```python
from build123d import *

# Parameters (mm, degrees)
SKETCH1_R           = 25
BOSS_EXTRUDE1_DEPTH = 20
SKETCH2_R           = 5
BOSS_EXTRUDE2_DEPTH = 10
SKETCH3_R           = 10
CUT_EXTRUDE1_DEPTH  = 41.620192023
CUT_EXTRUDE2_START  = -9
SKETCH5_R           = 25
SKETCH5_R_2         = 22.5
CUT_EXTRUDE2_DEPTH  = 8


with BuildPart() as part:
    # Sketch1 → Boss-Extrude1 (new body)
    with BuildSketch(Plane.XY):
        Circle(SKETCH1_R)
    extrude(amount=BOSS_EXTRUDE1_DEPTH)

    # Sketch2 → Boss-Extrude2 (add)
    with BuildSketch(Plane(origin=(0, 0, 0), x_dir=(-1, 0, 0), z_dir=(0, 0, -1))):
        with Locations(Location((0, -20, 0), (0, 0, 270))):
            Circle(SKETCH2_R)
    extrude(amount=BOSS_EXTRUDE2_DEPTH)

    # Sketch3 → Cut-Extrude1 (cut, through all)
    with BuildSketch(Plane(origin=(0, 0, 0), x_dir=(-1, 0, 0), z_dir=(0, 0, -1))):
        Circle(SKETCH3_R)
    extrude(amount=-CUT_EXTRUDE1_DEPTH, mode=Mode.SUBTRACT)

    # Sketch5 → Cut-Extrude2 (cut)
    with BuildSketch(Plane.XY.offset(20).offset(CUT_EXTRUDE2_START)):
        with Locations(Location((0, 0, 0), (0, 0, 270))):
            Circle(SKETCH5_R)
        Circle(SKETCH5_R_2, mode=Mode.SUBTRACT)
    extrude(amount=CUT_EXTRUDE2_DEPTH, mode=Mode.SUBTRACT)


solid = part.part
```
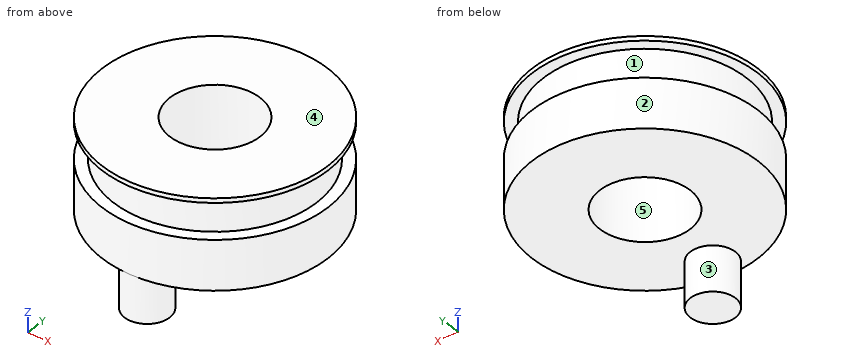
Geometry check sheet. Reference: the model listing, model coordinates, mm. Face numbers are marked on the shaded views. A direction names the side the tool comes from. Coordinates: 2 decimals unless noted, no trailing zeros. Order: outer loops, then holes, each group sorted by start corner. A loop starts at its lowest first (then second) coordinate and runs counter-clockwise, first axis right, second up. Notation, with made-up numbers: (-32.5, 82.5) - (9.5, 82.5) arc R33 cw to (9.5, 121.5) - close; hole circle Ø11 at (11, 18). An arc over 180 degrees is marked (long way). Use one line per item in the form item = value.
1. Section check D-D (x = 15). Record the boundary of the cut face in (y, z), then the cut area to 3 significant figures.
Here are the results:
outline = (-20, 0) - (20, 0) - (20, 11) - (16.77, 11) - (16.77, 19) - (20, 19) - (20, 20) - (-20, 20) - (-20, 19) - (-16.77, 19) - (-16.77, 11) - (-20, 11) - close
area = 748 mm²
2. Access from +Z, -Z, +X, -X, +Y, -Y to the whole of each face (thin tool, end or side, straight path). Record for the marked faces 1 and 2.
Here are the results:
face_1 = none
face_2 = +Z, -Z
3. Scan lines: line 1 (Y direction, x = 0, z = 7.25); line 2 (Z direction, x = -16.5, y = -15.5); line 3 (Z direction, x = -11.5, y = -9.5). Record each from-to range of solid material in increasing order.
Here are the results:
line_1 = -25 to -10, 10 to 25
line_2 = 0 to 11, 19 to 20
line_3 = 0 to 20
4. Draft check along Y on the marked faces 3, 4 and 5. Enter one of: pulls with the +Y half, pulls with the -Y half, needs draft (parallel to the pull), parting line crosses it, or undercut.
Here are the results:
face_3 = parting line crosses it
face_4 = needs draft
face_5 = undercut
5. Gauge pin test, flat ends, axial feed: pin 1 (3 mm diameter, centred on x = 8, z = 8.5, fed in from +Y); pin 2 (1.5 mm diameter, centred on y = 13.5, z = 12, fed in from +X); pin 3 (6 mm diameter, centred on y = -5.5, z = 15, fed in from -X). Record the tip position at first contact, or that the pin passes through.
Here are the results:
pin_1 = 24.14
pin_2 = 18.54
pin_3 = -22.36
6. Section check C-C (z = 3.25). Record the boundary of the cut face in (x, y), then the cut area to 3 significant figures.
Here are the results:
outline = circle Ø50 at (0, 0); hole circle Ø20 at (0, 0)
area = 1,650 mm²
7. Section check A-A (y = 0). Record the boundary of the cut face in (x, z), then the cut area to 3 significant figures.
Here are the results:
outline = (-25, 0) - (-10, 0) - (-10, 20) - (-25, 20) - (-25, 19) - (-22.5, 19) - (-22.5, 11) - (-25, 11) - close; (10, 0) - (25, 0) - (25, 11) - (22.5, 11) - (22.5, 19) - (25, 19) - (25, 20) - (10, 20) - close
area = 560 mm²
8. Section check B-B (x = -8). Record the boundary of the cut face in (y, z).
Here are the results:
outline = (-23.69, 0) - (-6, 0) - (-6, 20) - (-23.69, 20) - (-23.69, 19) - (-21.03, 19) - (-21.03, 11) - (-23.69, 11) - close; (6, 0) - (23.69, 0) - (23.69, 11) - (21.03, 11) - (21.03, 19) - (23.69, 19) - (23.69, 20) - (6, 20) - close
